from build123d import *

# Parameters (mm, degrees)
SKETCH1_R           = 73
BOSS_EXTRUDE1_DEPTH = 4
SKETCH2_R           = 73
SKETCH2_R_2         = 70
SKETCH2_R_3         = 68
SKETCH2_R_4         = 66
BOSS_EXTRUDE2_DEPTH = 6
CUT_EXTRUDE1_REACH  = 105.721
SKETCH4_W           = 30
SKETCH4_H           = 30
FILLET1_R           = 10
FILLET2_R           = 10
CUT_EXTRUDE2_REACH  = 105.721
SKETCH6_R           = 3


with BuildPart() as part:
    # Sketch1 → Boss-Extrude1 (new body)
    with BuildSketch(Plane(origin=(0, 0, 0), x_dir=(1, 0, 0), z_dir=(0, 1, 0))):
        with Locations(Location((0, 0, 0), (0, 0, 270))):
            Circle(SKETCH1_R)
    extrude(amount=BOSS_EXTRUDE1_DEPTH)

    # Sketch2 → Boss-Extrude2 (add)
    with BuildSketch(Plane(origin=(0, 4, 0), x_dir=(1, 0, 0), z_dir=(0, 1, 0))):
        with Locations(Location((0, 0, 0), (0, 0, 270))):
            Circle(SKETCH2_R)
        with Locations(Location((0, 0, 0), (0, 0, 270))):
            Circle(SKETCH2_R_2, mode=Mode.SUBTRACT)
        with Locations(Location((0, 0, 0), (0, 0, 270))):
            Circle(SKETCH2_R_3)
        with Locations(Location((0, 0, 0), (0, 0, 270))):
            Circle(SKETCH2_R_4, mode=Mode.SUBTRACT)
    extrude(amount=BOSS_EXTRUDE2_DEPTH)

    # Sketch4 → Cut-Extrude1 (cut, up to next)
    with BuildSketch(Plane.XZ, mode=Mode.PRIVATE) as cut_extrude1_sk1:
        with Locations((0, 58)):
            Rectangle(SKETCH4_W, SKETCH4_H)
    cut_extrude1_tool1 = extrude(cut_extrude1_sk1.sketch, amount=-CUT_EXTRUDE1_REACH, mode=Mode.PRIVATE) & part.part
    add(cut_extrude1_tool1.solids().sort_by_distance((0, 0, 58))[0], mode=Mode.SUBTRACT)

    # Fillet1
    fillet1_edges = [part.edges().sort_by_distance(p)[0] for p in [
        (15, 5, 71.442284398),
        (-15, 5, 71.442284398),
    ]]
    fillet(fillet1_edges, radius=FILLET1_R)

    # Fillet2
    fillet2_edges = [part.edges().sort_by_distance(p)[0] for p in [
        (-15, 2, 43),
        (15, 2, 43),
    ]]
    fillet(fillet2_edges, radius=FILLET2_R)

    # Sketch6 → Cut-Extrude2 (cut, up to next)
    with BuildSketch(Plane.XZ, mode=Mode.PRIVATE) as cut_extrude2_sk1:
        with Locations(Location((-60, 10, 0), (0, 0, 270))):
            Circle(SKETCH6_R)
    cut_extrude2_tool1 = extrude(cut_extrude2_sk1.sketch, amount=-CUT_EXTRUDE2_REACH, mode=Mode.PRIVATE) & part.part
    add(cut_extrude2_tool1.solids().sort_by_distance((-60, 0, 10))[0], mode=Mode.SUBTRACT)


solid = part.part
Could you check a few things on this model? Use its own coordinates, in mm. A direction names the side the tool comes from. Round coordinates to 2 decimals unless told otherwise and drop trailing zeros. Write each loop counter-clockwise with the first axis right and the second up, starting at its lowest first coordinate (ties: lowest second). Pieces come first, ordered by that corner, then holes. Notation, with made-up numbers: (56, -4) -> (112, -4) arc R29 cw to (112, 33) -> close; hole circle Ø6 at (17.25, -15). An arc over 180 degrees is marked (long way). Use a Markdown table: item, result.
1. We'd pull the mould along Z, two halves only. Please class faces 1 (the face through (61, 10, -26)), 2 (the face through (-57, 2, 10)), 3 (the face through (-11.99, 2.03, 45.85)), 4 (the face through (2.784, 6.958, -69.945)): +Z half, -Z half, draft (parallel to the pull), parting line (faces both ways), or undercut.
Answer key:
| item | result |
|---|---|
| face 1 | draft |
| face 2 | undercut |
| face 3 | +Z half |
| face 4 | undercut |
2. If we section it at B-B (z = 0): List the corners of the cut face in (x, y) for me, then the cut area to 3 significant figures.
Answer key:
| item | result |
|---|---|
| outline | (-73, 0) -> (73, 0) -> (73, 10) -> (70, 10) -> (70, 4) -> (68, 4) -> (68, 10) -> (66, 10) -> (66, 4) -> (-66, 4) -> (-66, 10) -> (-68, 10) -> (-68, 4) -> (-70, 4) -> (-70, 10) -> (-73, 10) -> close |
| area | 644 mm^2 |
3. If we section it at A-A (y = 1.5): List the corners of the cut face in (x, z) for me, then the cut area to 3 significant figures.
Answer key:
| item | result |
|---|---|
| outline | (-28.97, 67.01) arc R73 ccw (long way) to (28.97, 67.01) arc R10 ccw to (15, 57.83) -> (15, 53) arc R10 cw to (5, 43) -> (-5, 43) arc R10 cw to (-15, 53) -> (-15, 57.83) arc R10 ccw to start; hole circle Ø6 at (-60, 10) |
| area | 15,800 mm^2 |
4. Please list where these lines run through material, in increasing order: probe 1 along X at (y, z) = (7.5, 0); probe 2 along Z at (x, y) = (52, 5.5); probe 3 along Z at (x, y) = (-54, 5).
Answer key:
| item | result |
|---|---|
| probe 1 | x = -73 to -70, -68 to -66, 66 to 68, 70 to 73 |
| probe 2 | z = -51.23 to -46.86, -43.82 to -40.64, 40.64 to 43.82, 46.86 to 51.23 |
| probe 3 | z = -49.12 to -44.54, -41.33 to -37.95, 37.95 to 41.33, 44.54 to 49.12 |
5. Which directions (+Z, -Z, +X, -X, +Y, -Y) give clear straight access to the entire face, cutting with the end or side of a thin tool? Please do faces 5 (the face through (1, 4, -2)), 6 (the face through (1, 0, -4)), 7 (the face through (12.15, 2.03, 46.01)).
Answer key:
| item | result |
|---|---|
| face 5 | +Y |
| face 6 | +Z, -Z, +X, -X, -Y |
| face 7 | +Z, +Y, -Y |
6. If we section it at D-D (z = 48): List the corners of the cut face in (x, y) for me.
Answer key:
| item | result |
|---|---|
| outline | (-55, 0) -> (-13.66, 0) -> (-13.66, 4) -> (-45.3, 4) -> (-45.3, 10) -> (-48.17, 10) -> (-48.17, 4) -> (-50.95, 4) -> (-50.95, 10) -> (-55, 10) -> close; (13.66, 0) -> (55, 0) -> (55, 10) -> (50.95, 10) -> (50.95, 4) -> (48.17, 4) -> (48.17, 10) -> (45.3, 10) -> (45.3, 4) -> (13.66, 4) -> close |
7. For pin 1 Ø2 at (y, z) = (3, 55) entering from +X; pin 2 Ø8 at (x, z) = (-31, 12) entering from -Y; pin 3 Ø2 at (x, y) = (-16, 8) entering from -Z; pin 4 Ø4.5 at (x, y) = (-1.5, 2.5) entering from +Z, each with a flat end and sliding along its axis, tell me the tip position at first contact or that it passes through.
Answer key:
| item | result |
|---|---|
| pin 1 | stops at x = 49.12 |
| pin 2 | stops at y = 0 |
| pin 3 | stops at z = -71.44 |
| pin 4 | stops at z = 43 |
8. If we section it at C-C (x = 0): List the corners of the cut face in (y, z) for me.
Answer key:
| item | result |
|---|---|
| outline | (0, -73) -> (10, -73) -> (10, -70) -> (4, -70) -> (4, -68) -> (10, -68) -> (10, -66) -> (4, -66) -> (4, 43) -> (0, 43) -> close |
